Read the model definition and answer for the solid it produces. Units are mm, in the model's axes. Face numbers are marked on the shaded views. A direction names the side the tool comes from. Give positions to 0.01 mm unless a question says otherwise; leave off trailing zeros. Write each loop counter-clockwise with the first axis right and the second up, starting at its lowest first coordinate (ties: lowest second). Pieces come first, ordered by that corner, then holes. Notation, with made-up numbers: (-34, 78.25) - (-30, 78.25) arc R16 cw to (-30, 86.25) - close; hole circle Ø2 at (-36, 41). An arc over 180 degrees is marked (long way). Answer as a JSON object with one key per item and string values. Group by question number.
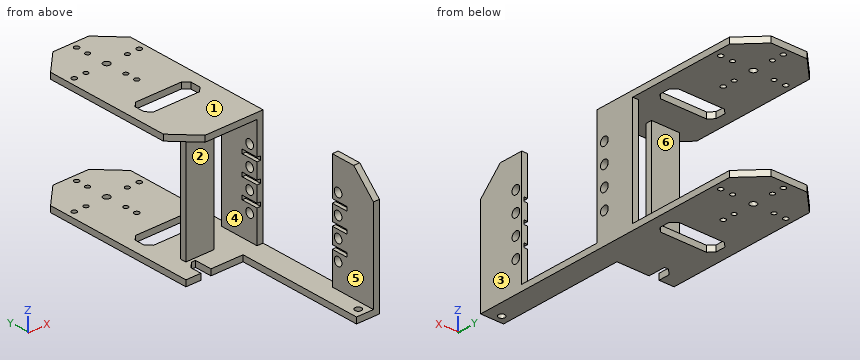
```python
from build123d import *

# Parameters (mm, degrees)
SKETCH_1_W           = 40
SKETCH_1_H           = 60
EXTRUDE_1_DEPTH      = 30
CHAMFER_3_SIZE       = 11
SKETCH_6_W           = 40
SKETCH_6_H           = 54
CUT_EXTRUDE_4_DEPTH  = 80
SKETCH_7_R           = 1.7
CUT_EXTRUDE_5_DEPTH  = 80
SKETCH_9_R           = 1.25
SKETCH_9_R_2         = 1.15
CUT_EXTRUDE_6_DEPTH  = 80
SKETCH_10_W          = 40
SKETCH_10_H          = 3
EXTRUDE_2_DEPTH      = 90
SKETCH_11_W          = 3
SKETCH_11_H          = 20
EXTRUDE_3_DEPTH      = 54
SKETCH_13_W          = 3
SKETCH_13_H          = 27.7
EXTRUDE_4_DEPTH      = 54
SKETCH_12_R          = 2.15
CUT_EXTRUDE_7_DEPTH  = 10
SKETCH_15_W          = 40
SKETCH_15_H          = 42
CUT_EXTRUDE_8_DEPTH  = 80
SKETCH_16_W          = 37
SKETCH_16_H          = 23
CUT_EXTRUDE_9_DEPTH  = 40
SKETCH_17_W          = 2
SKETCH_17_H          = 8.3
CUT_EXTRUDE_10_DEPTH = 1.8
SKETCH_18_W          = 54
SKETCH_18_H          = 3
EXTRUDE_5_DEPTH      = 28
SKETCH_19_W          = 14
SKETCH_19_H          = 54
CUT_EXTRUDE_11_DEPTH = 11.5
CHAMFER_4_SIZE       = 11
SKETCH_24_R          = 1.7
CUT_EXTRUDE_12_DEPTH = 35
SKETCH_25_R          = 1.65
CUT_EXTRUDE_13_DEPTH = 35
CUT_EXTRUDE_14_DEPTH = 65
CUT_EXTRUDE_15_DEPTH = 45
SKETCH_29_W          = 33.502223789
SKETCH_29_H          = 63.386780399
CUT_EXTRUDE_16_DEPTH = 10


with BuildPart() as part:
    # Sketch 1 → Extrude 1 (new, symmetric)
    with BuildSketch(Plane.XY):
        Rectangle(SKETCH_1_W, SKETCH_1_H)
    extrude(amount=EXTRUDE_1_DEPTH, both=True)

    # Chamfer 3
    chamfer_3_edges = [part.edges().sort_by_distance(p)[0] for p in [
        (-20, 30, 0),
        (20, 30, 0),
    ]]
    chamfer(chamfer_3_edges, length=CHAMFER_3_SIZE)

    # Sketch 6 → Cut-Extrude 4 (cut)
    with BuildSketch(Plane(origin=(0, 30, 0), x_dir=(1, 0, 0), z_dir=(0, 1, 0))):
        Rectangle(SKETCH_6_W, SKETCH_6_H)
    extrude(amount=-CUT_EXTRUDE_4_DEPTH, mode=Mode.SUBTRACT)


with BuildPart() as cut_extrude_4_piece_1:
    # of the separate pieces the step leaves, piece 1, a body of its own (cut_extrude_4_pieces)
    add(part.part.solids().sort_by_distance((-20, 19, -27))[0])


with BuildPart() as cut_extrude_4_piece_2:
    # of the separate pieces the step leaves, piece 2, a body of its own (cut_extrude_4_pieces)
    add(part.part.solids().sort_by_distance((-20, 19, 30))[0])


with BuildPart() as cut_extrude_5_tool:
    # Sketch 7 → Cut-Extrude 5 (new body)
    with BuildSketch(Plane.XY.offset(30)):
        with Locations((0, 10)):
            Circle(SKETCH_7_R)
    extrude(amount=-CUT_EXTRUDE_5_DEPTH)


with BuildPart() as cut_extrude_4_piece_1_1:
    add(cut_extrude_4_piece_1.part)

    # Cut-Extrude 5: cut by cut_extrude_5_tool
    add(cut_extrude_5_tool.part, mode=Mode.SUBTRACT)


with BuildPart() as cut_extrude_4_piece_2_1:
    add(cut_extrude_4_piece_2.part)

    # Cut-Extrude 5: cut by cut_extrude_5_tool
    add(cut_extrude_5_tool.part, mode=Mode.SUBTRACT)


with BuildPart() as cut_extrude_6_tool:
    # Sketch 9 → Cut-Extrude 6 (new body)
    with BuildSketch(Plane.XY.offset(30)):
        with Locations((-16.497956308, 9.740312384)):
            Circle(SKETCH_9_R)
        with Locations((-10.498699469, 9.834744245)):
            Circle(SKETCH_9_R_2)
        with Locations((-0.165255755, 20.498699469)):
            Circle(SKETCH_9_R_2)
        with Locations((-0.259687616, 26.497956308)):
            Circle(SKETCH_9_R)
        with Locations((10.498699469, 10.165255755)):
            Circle(SKETCH_9_R_2)
        with Locations((16.497956308, 10.259687616)):
            Circle(SKETCH_9_R)
        with Locations((0.165255755, -0.498699469)):
            Circle(SKETCH_9_R_2)
        with Locations((0.259687616, -6.497956308)):
            Circle(SKETCH_9_R)
    extrude(amount=-CUT_EXTRUDE_6_DEPTH)


with BuildPart() as cut_extrude_4_piece_1_2:
    add(cut_extrude_4_piece_1_1.part)

    # Cut-Extrude 6: cut by cut_extrude_6_tool
    add(cut_extrude_6_tool.part, mode=Mode.SUBTRACT)



with BuildPart() as cut_extrude_4_piece_2_2:
    add(cut_extrude_4_piece_2_1.part)

    # Cut-Extrude 6: cut by cut_extrude_6_tool
    add(cut_extrude_6_tool.part, mode=Mode.SUBTRACT)


with BuildPart() as cut_extrude_4_piece_1_3:
    add(cut_extrude_4_piece_1_2.part)

    add(cut_extrude_4_piece_2_2.part)  # Extrude 2 merges Cut-Extrude 4 piece 2
    # Sketch 10 → Extrude 2 (add)
    with BuildSketch(Plane.XZ.offset(30)):
        with Locations((0, 28.5)):
            Rectangle(SKETCH_10_W, SKETCH_10_H)
        with Locations((0, -28.5)):
            Rectangle(SKETCH_10_W, SKETCH_10_H)
    extrude(amount=EXTRUDE_2_DEPTH)

    # Sketch 11 → Extrude 3 (add)
    with BuildSketch(Plane.XY.offset(-27)):
        with Locations((18.5, -45)):
            Rectangle(SKETCH_11_W, SKETCH_11_H)
    extrude(amount=EXTRUDE_3_DEPTH)

    # Sketch 13 → Extrude 4 (add)
    with BuildSketch(Plane.XY.offset(-27)):
        with Locations((18.5, -106.15)):
            Rectangle(SKETCH_13_W, SKETCH_13_H)
    extrude(amount=EXTRUDE_4_DEPTH)

    # Sketch 12 → Cut-Extrude 7 (cut)
    with BuildSketch(Plane(origin=(20, 0, 0), x_dir=(0, 0, -1), z_dir=(1, 0, 0))):
        with Locations((-14.775, -50.85)):
            Circle(SKETCH_12_R)
        with Locations((-4.925, -50.85)):
            Circle(SKETCH_12_R)
        with Locations((-14.775, -100.27)):
            Circle(SKETCH_12_R)
        with Locations((-4.925, -100.27)):
            Circle(SKETCH_12_R)
        with Locations((4.925, -100.27)):
            Circle(SKETCH_12_R)
        with Locations((14.775, -100.27)):
            Circle(SKETCH_12_R)
        with Locations(Location((4.925, -50.85, 0), (0, 0, 90))):
            Circle(SKETCH_12_R)
        with Locations(Location((14.775, -50.85, 0), (0, 0, 90))):
            Circle(SKETCH_12_R)
    extrude(amount=-CUT_EXTRUDE_7_DEPTH, mode=Mode.SUBTRACT)

    # Sketch 15 → Cut-Extrude 8 (cut)
    with BuildSketch(Plane.XY.offset(-27)):
        with Locations((0, -76)):
            Rectangle(SKETCH_15_W, SKETCH_15_H)
    extrude(amount=CUT_EXTRUDE_8_DEPTH, mode=Mode.SUBTRACT)

    # Sketch 16 → Cut-Extrude 9 (cut)
    with BuildSketch(Plane(origin=(0, 0, 27), x_dir=(-1, 0, 0), z_dir=(0, 0, -1))):
        with Locations((1.5, -108.5)):
            Rectangle(SKETCH_16_W, SKETCH_16_H)
    extrude(amount=-CUT_EXTRUDE_9_DEPTH, mode=Mode.SUBTRACT)

    # Sketch 17 → Cut-Extrude 10 (cut)
    with BuildSketch(Plane.ZY.offset(-17)):
        with Locations((0, -50.85)):
            Rectangle(SKETCH_17_W, SKETCH_17_H)
        with Locations((-9.85, -50.85)):
            Rectangle(SKETCH_17_W, SKETCH_17_H)
        with Locations((9.85, -50.85)):
            Rectangle(SKETCH_17_W, SKETCH_17_H)
        with Locations((9.85, -101.15)):
            Rectangle(SKETCH_17_W, SKETCH_17_H)
        with Locations((-9.85, -101.15)):
            Rectangle(SKETCH_17_W, SKETCH_17_H)
        with Locations((0, -101.15)):
            Rectangle(SKETCH_17_W, SKETCH_17_H)
    extrude(amount=-CUT_EXTRUDE_10_DEPTH, mode=Mode.SUBTRACT)

    # Sketch 18 → Extrude 5 (add)
    with BuildSketch(Plane.ZY.offset(-17)):
        with Locations((0, -45)):
            Rectangle(SKETCH_18_W, SKETCH_18_H)
    extrude(amount=EXTRUDE_5_DEPTH)

    # Sketch 19 → Cut-Extrude 11 (cut)
    with BuildSketch(Plane(origin=(0, -43.5, 0), x_dir=(1, 0, 0), z_dir=(0, 1, 0))):
        with Locations((10, 0)):
            Rectangle(SKETCH_19_W, SKETCH_19_H)
    extrude(amount=-CUT_EXTRUDE_11_DEPTH, mode=Mode.SUBTRACT)

    # Chamfer 4
    chamfer_4_edges = [cut_extrude_4_piece_1_3.edges().sort_by_distance(p)[0] for p in [
        (-20, -55, 28.5),
        (18.5, -120, 30),
        (-20, -120, -28.5),
    ]]
    chamfer(chamfer_4_edges, length=CHAMFER_4_SIZE)

    # Sketch 24 → Cut-Extrude 12 (cut)
    with BuildSketch(Plane.XY.offset(-27)):
        with Locations((-14, -79)):
            Circle(SKETCH_24_R)
        with Locations((-14, -89)):
            Circle(SKETCH_24_R)
    extrude(amount=-CUT_EXTRUDE_12_DEPTH, mode=Mode.SUBTRACT)

    # Sketch 25 → Cut-Extrude 13 (cut)
    with BuildSketch(Plane.XY.offset(-27)):
        with Locations((3, -116)):
            Circle(SKETCH_25_R)
        with Locations((13, -116)):
            Circle(SKETCH_25_R)
    extrude(amount=-CUT_EXTRUDE_13_DEPTH, mode=Mode.SUBTRACT)

    # Sketch 27 → Cut-Extrude 14 (cut)
    with BuildSketch(Plane(origin=(0, 0, -30), x_dir=(-1, 0, 0), z_dir=(0, 0, -1))):
        Polygon((-14, -21.5), (-11.5, -19), (11.5, -19), (14, -21.5), (14, -26.5), (11.5, -29), (-11.5, -29), (-14, -26.5), align=None)
    extrude(amount=-CUT_EXTRUDE_14_DEPTH, mode=Mode.SUBTRACT)

    # Sketch 28 → Cut-Extrude 15 (cut)
    with BuildSketch(Plane(origin=(0, 0, -30), x_dir=(-1, 0, 0), z_dir=(0, 0, -1))):
        Polygon((-4, -105), (-1, -105), (-1, -81), (-4, -81), (-7, -84), (-7, -102), align=None)
        Polygon((7.5, -70), (9.5, -70), (12.5, -67), (12.5, -51), (9.5, -48), (7.5, -48), align=None)
    extrude(amount=-CUT_EXTRUDE_15_DEPTH, mode=Mode.SUBTRACT)

    # Sketch 29 → Cut-Extrude 16 (cut)
    with BuildSketch(Plane.XY.offset(-27)):
        with Locations((-8.200271599, -88.306609801)):
            Rectangle(SKETCH_29_W, SKETCH_29_H)
    extrude(amount=-CUT_EXTRUDE_16_DEPTH, mode=Mode.SUBTRACT)


solid = cut_extrude_4_piece_1_3.part
```
1) Flat-ended cylindrical pins translate along their axes: pin 1 Ø1.8 at (x, y) = (-0.17, 20.5) entering from +Z; pin 2 Ø1.6 at (y, z) = (-101, 0) entering from -X; pin 3 Ø1.6 at (x, z) = (-8, -28.5) entering from -Y; pin 4 Ø12 at (x, z) = (12.5, 15) entering from +Y. Find the tip coordinate at first contact, or state that the pin passes through.
2) Find section B-B, the plane y = -100.27. Give the number of separate pieces and of enclosed holes in the cut face, and give its area (3 significant figures).
3) For a pull along X with two mould halves and no side action, classify the marked faces 3, 4, 5 and 6 as released by +X, released by -X, zero draft, split by the parting line, or undercut.
4) Find section C-C, the plane y = -116. Write down the section's boundary in (x, z), and give its area (3 significant figures).
5) Which of the six approach directions +Z, -Z, +X, -X, +Y, -Y give full straight-line access (tool end or side, diameter ignored) to the marked faces 1 and 2?
6) Find the intervals of material crossed by line 1 (Y direction, x = 18, z = 2); line 2 (Z direction, x = -6.5, y = -9); line 3 (Y direction, x = -6, z = -6), in increasing order. Write a range as [from, to].
7) Find section A-A, the plane z = -18.5. Write down the section's boundary in (x, y).
Values follow:
{
 "1": {"pin 1": "passes through", "pin 2": "stops at x = 18.8", "pin 3": "stops at y = -56.61", "pin 4": "stops at y = -35"},
 "2": {"separate pieces": "5", "enclosed holes": "0", "area": "143 mm2"},
 "3": {"face 3": "released by +X", "face 4": "undercut", "face 5": "released by -X", "face 6": "zero draft"},
 "4": {"outline": "(8.55, -30) - (11.35, -30) - (11.35, -27) - (8.55, -27) - close; (14.65, -30) - (20, -30) - (20, 23) - (17, 23) - (17, -27) - (14.65, -27) - close", "area": "174 mm2"},
 "5": {"face 1": "+Z, +X, -X, +Y, -Y", "face 2": "-X, -Y"},
 "6": {"line 1": "y = [-120, -97], [-55, -35]", "line 2": "z = [-30, -27], [27, 30]", "line 3": "y = [-46.5, -43.5]"},
 "7": {"outline": "(-11, -46.5) - (3, -46.5) - (3, -43.5) - (-11, -43.5) - close; (17, -120) - (20, -120) - (20, -97) - (17, -97) - close; (17, -55) - (20, -55) - (20, -35) - (17, -35) - close"}
}
